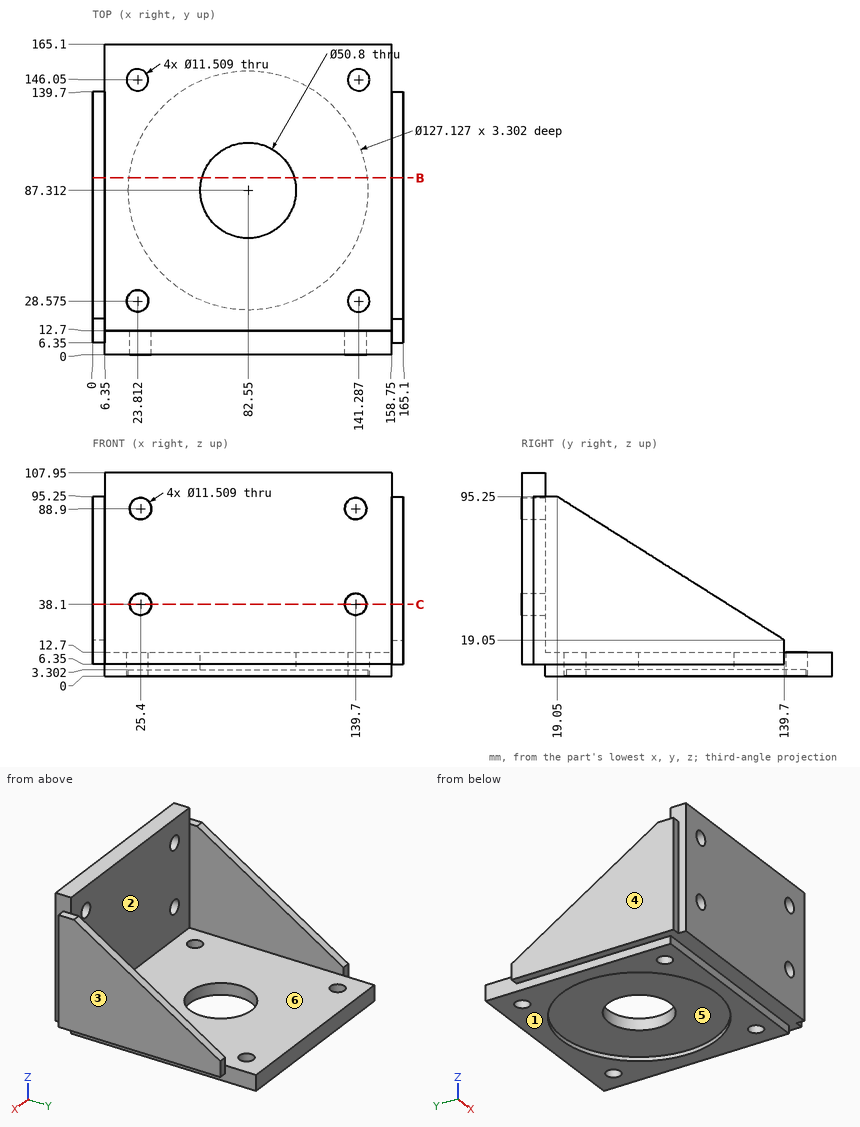
Design review of the part shown in the three views and the two pictorial views. Dimensions are in mm from the part's minimum x, y and z. A direction names the side the tool comes from. Round coordinates to 2 decimals unless told otherwise and drop trailing zeros. Loops run counter-clockwise (first coordinate to the right, second up) from the corner with the lowest first, then second, coordinate; pieces in that order, holes last. Notation, with made-up numbers: (45, 79.5) - (71, 79.5) arc R32 ccw to (71, 111.5) - close; hole circle Ø11 at (1.5, 67). An arc over 180 degrees is marked (long way). One line per item, written item: value. Start each with the question number.
Item 1: The part is to be moulded in two halves that separate along X. For the marked faces 1, 2 and 3, say which applies: +X half, -X half, draft (parallel to the pull), parting line (faces both ways), or undercut.
Item 2: Take a section at C-C (z = 38.1). State how many separate pieces and enclosed holes the cut face has, plus the area to 3 significant figures.
Item 3: Clearance check with flat-ended pins moving along their axes: pin 1 Ø4 at (x, z) = (144.5, 56) entering from +Y; pin 2 Ø15 at (x, y) = (141.29, 146.05) entering from +Z; pin 3 Ø1.9 at (x, z) = (2, 45.5) entering from -Y; pin 4 Ø3 at (x, z) = (130, 74.5) entering from -Y. State where each tip first meets the part, or that it passes through.
Item 4: For L1, parallel to X at y = 7.5, z = 38.1 (1 decimal); L2, parallel to X at y = 146.05, z = 4; L3, parallel to Z at x = 139, y = 7, list the stretches that pass through material, from the lowest coordinate up.
Item 5: Take a section at B-B (y = 94). Give the boundary of the cut face in (x, z).
Item 6: For the marked faces 4, 5 and 6, list the 3-axis set-ups (+Z, -Z, +X, -X, +Y, -Y) from which the entire face can be reached by the end or side of a thin tool; tool diameter is ignored.
Answer below:
1. face 1: draft
1. face 2: undercut
1. face 3: +X half
2. separate pieces: 3
2. enclosed holes: 0
2. area: 2,950 mm2
3. pin 1: stops at y = 12.7
3. pin 2: stops at z = 12.7
3. pin 3: stops at y = 6.35
3. pin 4: stops at y = 0
4. L1: x = 0 to 19.6, 31.2 to 133.9, 145.5 to 165.1
4. L2: x = 6.35 to 18.06, 29.57 to 135.53, 147.04 to 158.75
4. L3: z = 6.35 to 32.39, 43.81 to 83.19, 94.61 to 107.95
5. outline: (0, 6.35) - (6.35, 6.35) - (6.35, 0) - (19.34, 0) - (19.34, 3.3) - (58.05, 3.3) - (58.05, 12.7) - (6.35, 12.7) - (6.35, 47.91) - (0, 47.91) - close; (107.05, 3.3) - (145.76, 3.3) - (145.76, 0) - (158.75, 0) - (158.75, 6.35) - (165.1, 6.35) - (165.1, 47.91) - (158.75, 47.91) - (158.75, 12.7) - (107.05, 12.7) - close
6. face 4: +Z, -Z, -X, +Y, -Y
6. face 5: -Z
6. face 6: +Z, +Y
